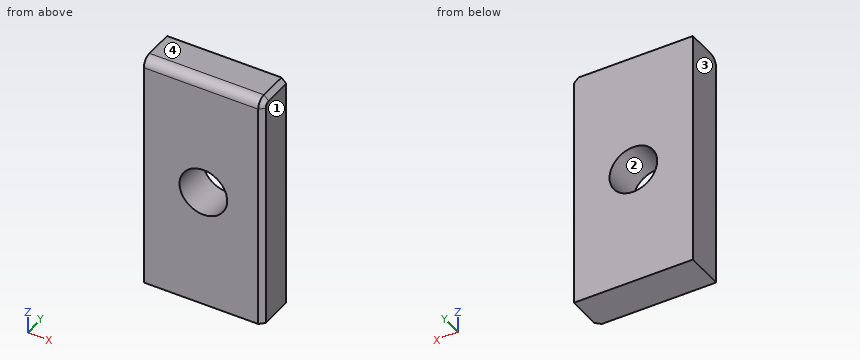
from build123d import *

# Parameters (mm, degrees)
F0_W     = 127
F0_H     = 254
F0_R     = 25.4
F1_DEPTH = 40.894
F2_R     = 10
F3_SIZE  = 5


with BuildPart() as f1:
    # F0 (on Front) → F1 (new body)
    with BuildSketch(Plane.XZ):
        Rectangle(F0_W, F0_H)
        Circle(F0_R, mode=Mode.SUBTRACT)
    extrude(amount=F1_DEPTH)

    # F2
    f2_edges = [f1.edges().sort_by_distance(p)[0] for p in [
        (0, -40.894, 127),
    ]]
    fillet(f2_edges, radius=F2_R)

    # F3
    f3_edges = [f1.edges().sort_by_distance(p)[0] for p in [
        (63.5, -40.894, -5),
    ]]
    chamfer(f3_edges, length=F3_SIZE)


solid = f1.part
Can you work these out from the model? Positions are in its coordinate system, mm. Face numbers are marked on the shaded views. Give positions to 0.01 mm unless a question says otherwise; leave off trailing zeros. Write each loop counter-clockwise with the first axis right and the second up, starting at its lowest first coordinate (ties: lowest second). Pieces come first, ordered by that corner, then holes. Notation, with made-up numbers: (-22.75, -13) -> (-18.75, -13) arc R20 ccw to (-18.75, 24) -> close; hole circle Ø4 at (25, -33). An arc over 180 degrees is marked (long way). Answer as a JSON object with one key per item and string values. Group by question number.
Item 1: Suppose I cut it at C-C (y = -23.5). Please give me the cut outline in (x, z).
Item 2: Please list where these lines run through material, in increasing order: line 1 (Z direction, x = 0, y = -12); line 2 (X direction, y = -5, z = 0.5); line 3 (Z direction, x = 4, y = -31). Write a range as [from, to].
Item 3: Suppose I cut it at B-B (z = 0). Please give me the cut outline in (x, y).
Item 4: Suppose I cut it at A-A (x = 0). Please give me the cut outline in (y, z).
Item 5: We'd pull the mould along X, two halves only. Please class the marked faces 1, 2, 3 and 4: +X half, -X half, draft (parallel to the pull), parting line (faces both ways), or undercut.
Findings:
{
 "1": {"outline": "(-63.5, -127) -> (63.5, -127) -> (63.5, 122) -> (58.5, 127) -> (-63.5, 127) -> close; hole circle Ø50.8 at (0, 0)"},
 "2": {"line 1": "z = [-127, -25.4], [25.4, 127]", "line 2": "x = [-63.5, -25.4], [25.4, 63.5]", "line 3": "z = [-127, -25.08], [25.08, 127]"},
 "3": {"outline": "(-63.5, -40.89) -> (-25.4, -40.89) -> (-25.4, 0) -> (-63.5, 0) -> close; (25.4, -40.89) -> (58.5, -40.89) -> (63.5, -35.89) -> (63.5, 0) -> (25.4, 0) -> close"},
 "4": {"outline": "(-40.89, -127) -> (0, -127) -> (0, -25.4) -> (-40.89, -25.4) -> close; (-40.89, 25.4) -> (0, 25.4) -> (0, 127) -> (-30.89, 127) arc R10 ccw to (-40.89, 117) -> close"},
 "5": {"face 1": "+X half", "face 2": "undercut", "face 3": "-X half", "face 4": "draft"}
}
